Could you check a few things on this model? Use its own coordinates, in mm. A direction names the side the tool comes from. Round coordinates to 2 decimals unless told otherwise and drop trailing zeros. Write each loop counter-clockwise with the first axis right and the second up, starting at its lowest first coordinate (ties: lowest second). Pieces come first, ordered by that corner, then holes. Notation, with made-up numbers: (-30, -32.5) -> (21, -32.5) arc R19 cw to (21, -1.5) -> close; hole circle Ø2 at (36, -36). An arc over 180 degrees is marked (long way). Return JSON: item names as keys, results as strings.
from build123d import *

# Parameters (mm, degrees)
ESQUISSE1_R             = 1.15
ESQUISSE1_R_2           = 1.1
BOSS_EXTRU_1_DEPTH      = 1.8
ESQUISSE2_W             = 19
ESQUISSE2_H             = 26.8
BOSS_EXTRU_2_DEPTH      = 2
ESQUISSE3_W             = 4.5
ESQUISSE3_H             = 26.8
BOSS_EXTRU_3_DEPTH      = 0.01
ESQUISSE4_W             = 3.5
ESQUISSE4_H             = 1.5
ENL_V_MAT_EXTRU_1_DEPTH = 0.02
ESQUISSE5_W             = 12
ESQUISSE5_H             = 8
BOSS_EXTRU_4_DEPTH      = 5
ESQUISSE6_W             = 3
ESQUISSE6_H             = 1.5
ENL_V_MAT_EXTRU_2_DEPTH = 1
ESQUISSE8_W             = 4.6
ESQUISSE8_H             = 3.292306134
ENL_V_MAT_EXTRU_3_DEPTH = 1
CHANFREIN1_SIZE         = 1
ENL_V_MAT_EXTRU_4_DEPTH = 5
ESQUISSE10_W            = 1
ESQUISSE10_H            = 1
ENL_V_MAT_EXTRU_5_DEPTH = 4
ESQUISSE11_W            = 1
ESQUISSE11_H            = 1
ENL_V_MAT_EXTRU_7_DEPTH = 5
ESQUISSE12_R            = 2.25
BOSS_EXTRU_5_DEPTH      = 3.3


with BuildPart() as part:
    # Esquisse1 → Boss.-Extru.1 (new body)
    with BuildSketch(Plane.XY):
        with BuildLine():
            Line((-12.744645331, 10.992907801), (-12.744645331, 3.192907801))
            ThreePointArc((-12.744645331, 3.192907801), (-14.944645331, 0.992907801), (-12.744645331, -1.207092199))
            Line((-12.744645331, -1.207092199), (-12.744645331, -9.007092199))
            Line((-12.744645331, -9.007092199), (-4.994645331, -9.007092199))
            ThreePointArc((-4.994645331, -9.007092199), (-2.744645331, -6.757092199), (-0.494645331, -9.007092199))
            Line((-0.494645331, -9.007092199), (7.255354669, -9.007092199))
            Line((7.255354669, -9.007092199), (7.255354669, -1.207092199))
            ThreePointArc((7.255354669, -1.207092199), (9.455354669, 0.992907801), (7.255354669, 3.192907801))
            Line((7.255354669, 3.192907801), (7.255354669, 10.992907801))
            Line((7.255354669, 10.992907801), (7.255354669, 18.792907801))
            ThreePointArc((7.255354669, 18.792907801), (5.055354669, 20.992907801), (7.255354669, 23.192907801))
            Line((7.255354669, 23.192907801), (7.255354669, 30.992907801))
            Line((7.255354669, 30.992907801), (-0.744645331, 30.992907801))
            ThreePointArc((-0.744645331, 30.992907801), (-2.744645331, 32.992907801), (-4.744645331, 30.992907801))
            Line((-4.744645331, 30.992907801), (-12.744645331, 30.992907801))
            Line((-12.744645331, 30.992907801), (-12.744645331, 23.192907801))
            ThreePointArc((-12.744645331, 23.192907801), (-10.544645331, 20.992907801), (-12.744645331, 18.792907801))
            Line((-12.744645331, 18.792907801), (-12.744645331, 10.992907801))
        make_face()
        with Locations((-12.744645331, 0.992907801)):
            Circle(ESQUISSE1_R, mode=Mode.SUBTRACT)
        with Locations((7.255354669, 0.992907801)):
            Circle(ESQUISSE1_R, mode=Mode.SUBTRACT)
        with Locations((-2.744645331, 30.992907801)):
            Circle(ESQUISSE1_R_2, mode=Mode.SUBTRACT)
    extrude(amount=BOSS_EXTRU_1_DEPTH)

    # Esquisse2 → Boss.-Extru.2 (add)
    with BuildSketch(Plane.XY.offset(1.8)):
        with Locations((-2.744645331, 15.292907801)):
            Rectangle(ESQUISSE2_W, ESQUISSE2_H)
    extrude(amount=BOSS_EXTRU_2_DEPTH)

    # Esquisse3 → Boss.-Extru.3 (add)
    with BuildSketch(Plane.XY.offset(3.8)):
        with Locations((-9.994645331, 15.292907801)):
            Rectangle(ESQUISSE3_W, ESQUISSE3_H)
    extrude(amount=BOSS_EXTRU_3_DEPTH)

    # Esquisse4 → Enlèv. mat.-Extru.1 (cut)
    with BuildSketch(Plane.XY.offset(3.81)):
        with Locations((-9.494645331, 23.942907801)):
            Rectangle(ESQUISSE4_W, ESQUISSE4_H)
        with Locations((-9.494645331, 6.642907801)):
            Rectangle(ESQUISSE4_W, ESQUISSE4_H)
    extrude(amount=-ENL_V_MAT_EXTRU_1_DEPTH, mode=Mode.SUBTRACT)

    # Esquisse5 → Boss.-Extru.4 (add)
    with BuildSketch(Plane(origin=(0, 0, 0), x_dir=(-1, 0, 0), z_dir=(0, 0, -1))):
        with Locations((2.744645331, -4.138713158)):
            Rectangle(ESQUISSE5_W, ESQUISSE5_H)
    extrude(amount=BOSS_EXTRU_4_DEPTH)

    # Esquisse6 → Enlèv. mat.-Extru.2 (cut)
    with BuildSketch(Plane(origin=(0, 0, -5), x_dir=(-1, 0, 0), z_dir=(0, 0, -1))):
        Polygon((8.744645331, -0.138713158), (-3.255354669, -0.138713158), (-3.255354669, -1.038713158), (-0.555354669, -1.038713158), (-0.555354669, -8.138713158), (6.044645331, -8.138713158), (6.044645331, -1.038713158), (8.744645331, -1.038713158), align=None)
        with Locations((2.725727115, -4.088713158)):
            Rectangle(ESQUISSE6_W, ESQUISSE6_H, mode=Mode.SUBTRACT)
    extrude(amount=-ENL_V_MAT_EXTRU_2_DEPTH, mode=Mode.SUBTRACT)

    # Esquisse8 → Enlèv. mat.-Extru.3 (cut)
    with BuildSketch(Plane(origin=(0, 0, -4), x_dir=(-1, 0, 0), z_dir=(0, 0, -1))):
        with Locations((2.744645331, -6.492560091)):
            Rectangle(ESQUISSE8_W, ESQUISSE8_H)
    extrude(amount=-ENL_V_MAT_EXTRU_3_DEPTH, mode=Mode.SUBTRACT)

    # Chanfrein1
    chanfrein1_edges = [part.edges().sort_by_distance(p)[0] for p in [
        (-2.725727115, -4.838713158, -5),
    ]]
    chamfer(chanfrein1_edges, length=CHANFREIN1_SIZE - 0.0001)  # a hair under: the kernel refuses the full size

    # Esquisse9 → Enlèv. mat.-Extru.4 (cut)
    with BuildSketch(Plane.XZ.offset(8.138713158)):
        Polygon((-7.144645331, -0.7), (1.655354669, -0.7), (1.655354669, -3.7), (1.655354669, -4.5), (0.855354669, -4.5), (0.855354669, -3.7), (-6.344645331, -3.7), (-6.344645331, -4.5), (-7.144645331, -4.5), (-7.144645331, -3.7), align=None)
    extrude(amount=-ENL_V_MAT_EXTRU_4_DEPTH, mode=Mode.SUBTRACT)

    # Esquisse10 → Enlèv. mat.-Extru.5 (cut)
    with BuildSketch(Plane.XZ.offset(8.138713158)):
        with Locations((-8.244645331, -3.5)):
            Rectangle(ESQUISSE10_W, ESQUISSE10_H)
        with Locations((2.755354669, -3.5)):
            Rectangle(ESQUISSE10_W, ESQUISSE10_H)
    extrude(amount=-ENL_V_MAT_EXTRU_5_DEPTH, mode=Mode.SUBTRACT)

    # Esquisse11 → Enlèv. mat.-Extru.7 (cut)
    with BuildSketch(Plane(origin=(0, 0, -5), x_dir=(-1, 0, 0), z_dir=(0, 0, -1))):
        with Locations((-2.755354669, -7.638713158)):
            Rectangle(ESQUISSE11_W, ESQUISSE11_H)
        with Locations((8.244645331, -7.638713158)):
            Rectangle(ESQUISSE11_W, ESQUISSE11_H)
    extrude(amount=-ENL_V_MAT_EXTRU_7_DEPTH, mode=Mode.SUBTRACT)

    # Esquisse12 → Boss.-Extru.5 (add)
    with BuildSketch(Plane(origin=(0, 0, 0), x_dir=(-1, 0, 0), z_dir=(0, 0, -1))):
        with Locations(Location((2.744645331, 20.036668052, 0), (0, 0, 180))):
            Circle(ESQUISSE12_R)
    extrude(amount=BOSS_EXTRU_5_DEPTH)


solid = part.part
1) Thinking about a two-plate mould opening in X: for faces 6 (the face through (-8.3, -4.139, -3.5)), 7 (the face through (8.318, 0.552, 0.887)), 8 (the face through (-1.535, 18.139, -1.627)), 9 (the face through (-2.98, 29.92, 0.89)), which applies, pulls with the +X half, pulls with the -X half, needs draft (parallel to the pull), parting line crosses it, or undercut?
Return value:
{"face 6": "needs draft", "face 7": "undercut", "face 8": "parting line crosses it", "face 9": "undercut"}
2) If I drill on probe 1 along Z at (x, y) = (-2.75, -3.5); probe 2 along X at (y, z) = (12, 0.5); probe 3 along Z at (x, y) = (-6.75, 14), over which ranges is the centre line in solid material (lowest first)? Write a range as [from, to].
Return value:
{"probe 1": "[-5, -3.7], [-0.7, 1.8]", "probe 2": "[-12.74, 7.26]", "probe 3": "[0, 3.8]"}
3) I want a section at D-D, the plane x = 7.75. Please give me the cut outline in (y, z).
Return value:
{"outline": "(-1.15, 0) -> (-0.05, 0) -> (-0.05, 1.8) -> (-1.15, 1.8) -> close; (2.03, 0) -> (3.14, 0) -> (3.14, 1.8) -> (2.03, 1.8) -> close"}
4) For faces 1 (the face through (2.8, -7.139, -4.5)), 2 (the face through (-7.4, -1.039, -4.5)), 3 (the face through (-2.7, -3.339, -4.5)), 4 (the face through (-8, -6, -4)), 5 (the face through (5.056, 20.945, 0.887)), which set-ups out of +Z, -Z, +X, -X, +Y, -Y let a thin tool reach every point of the face, with its end or its side?
Return value:
{"face 1": "-Z, +X, -Y", "face 2": "-Z, +X, -X, +Y", "face 3": "-Z, +Y", "face 4": "-X, -Y", "face 5": "-Z, +X"}
5) I want a section at B-B, the plane z = -1.5. Please give me the cut outline in (x, y), and give its area (3 significant figures).
Return value:
{"outline": "(-8.74, -7.14) -> (-7.74, -7.14) -> (-7.74, -8.14) -> (-7.14, -8.14) -> (-7.14, -3.14) -> (1.66, -3.14) -> (1.66, -8.14) -> (2.26, -8.14) -> (2.26, -7.14) -> (3.26, -7.14) -> (3.26, -0.14) -> (-8.74, -0.14) -> close; circle Ø4.5 at (-2.74, 20.04)", "area": "65.9 mm²"}
6) Will these pins go through, and if not, where does the flat tip stop? pin 1 Ø1 at (x, y) = (-5.5, -1) entering from +Z; pin 2 Ø1.4 at (x, y) = (-12, 22) entering from -Z; pin 3 Ø12 at (x, y) = (4.5, -1.5) entering from +Z; pin 4 Ø5 at (x, z) = (-12.5, -3) entering from -Y.
Return value:
{"pin 1": "z = 1.8", "pin 2": "z = 1.8", "pin 3": "z = 3.8", "pin 4": "through"}
